Geometry check sheet. Reference: the model listing, model coordinates, mm. A direction names the side the tool comes from. Round coordinates to 2 decimals unless told otherwise and drop trailing zeros. Order: outer loops, then holes, each group sorted by start corner. A loop starts at its lowest first (then second) coordinate and runs counter-clockwise, first axis right, second up.
```python
from build123d import *

# Parameters (mm, degrees)
SKETCH2_R           = 145
SKETCH2_R_2         = 105
BOSS_EXTRUDE2_START = -50
SKETCH3_W           = 360
SKETCH3_H           = 360
SKETCH3_R           = 145
BOSS_EXTRUDE2_DEPTH = 50
FILLET4_R           = 20
SKETCH4_R           = 145
BOSS_EXTRUDE3_DEPTH = 50
SKETCH6_R           = 30
CUT_EXTRUDE1_DEPTH  = 10
CUT_EXTRUDE2_REACH  = 746.668
SKETCH7_R           = 15
CIRPATTERN1_COUNT   = 4
SKETCH9_R           = 30
CUT_EXTRUDE4_DEPTH  = 10
CUT_EXTRUDE5_REACH  = 866.02
SKETCH11_R          = 15
CIRPATTERN3_COUNT   = 4
CHAMFER1_SIZE       = 10


with BuildPart() as part:
    # Sweep-Thin1: sweep along a path in Sketch1
    with BuildLine(Plane.XY) as sweep_thin1_path:
        Line((0, 0), (-150, 0))
        ThreePointArc((-150, 0), (-333.847763109, 76.152236891), (-410, 260))
        Line((-410, 260), (-410, 410))
    # Sketch2 → Sweep-Thin1 (sweep)
    with BuildSketch(Plane(origin=(0, 0, 0), x_dir=(0, 0, -1), z_dir=(1, 0, 0))):
        Circle(SKETCH2_R)
        Circle(SKETCH2_R_2, mode=Mode.SUBTRACT)
    sweep(path=sweep_thin1_path.line)

    # Sketch3 → Boss-Extrude2 (add)
    with BuildSketch(Plane(origin=(0, 0, 0), x_dir=(0, 0, -1), z_dir=(1, 0, 0)).offset(BOSS_EXTRUDE2_START)):
        Rectangle(SKETCH3_W, SKETCH3_H)
        with Locations(Location((0, 0, 0), (0, 0, 270))):
            Circle(SKETCH3_R, mode=Mode.SUBTRACT)
    extrude(amount=BOSS_EXTRUDE2_DEPTH)

    # Fillet4
    fillet4_edges = [part.edges().sort_by_distance(p)[0] for p in [
        (-25, 180, -180),
        (-25, -180, -180),
        (-25, -180, 180),
        (-25, 180, 180),
    ]]
    fillet(fillet4_edges, radius=FILLET4_R)

    # Sketch4 → Boss-Extrude3 (add)
    with BuildSketch(Plane(origin=(0, 410, 0), x_dir=(1, 0, 0), z_dir=(0, 1, 0))):
        with BuildLine():
            Line((-255.005170931, 180), (-595.005170931, 180))
            ThreePointArc((-595.005170931, 180), (-602.076238742, 177.071067812), (-605.005170931, 170))
            Line((-605.005170931, 170), (-605.005170931, -170))
            ThreePointArc((-605.005170931, -170), (-602.076238742, -177.071067812), (-595.005170931, -180))
            Line((-595.005170931, -180), (-255.005170931, -180))
            ThreePointArc((-255.005170931, -180), (-247.934103119, -177.071067812), (-245.005170931, -170))
            Line((-245.005170931, -170), (-245.005170931, 170))
            ThreePointArc((-245.005170931, 170), (-247.934103119, 177.071067812), (-255.005170931, 180))
        make_face()
        with Locations(Location((-410, 0, 0), (0, 0, 180))):
            Circle(SKETCH4_R, mode=Mode.SUBTRACT)
    extrude(amount=-BOSS_EXTRUDE3_DEPTH)

    # Sketch6 → Cut-Extrude1 (cut)
    with BuildSketch(Plane(origin=(0, 0, 0), x_dir=(0, 0, -1), z_dir=(1, 0, 0))):
        with Locations((-130, 130)):
            Circle(SKETCH6_R)
    cut_extrude1 = extrude(amount=-CUT_EXTRUDE1_DEPTH, mode=Mode.SUBTRACT)

    # Sketch7 → Cut-Extrude2 (cut, up to next)
    with BuildSketch(Plane(origin=(-10, 0, 0), x_dir=(0, 0, -1), z_dir=(1, 0, 0)), mode=Mode.PRIVATE) as cut_extrude2_sk1:
        with Locations((-130, 130)):
            Circle(SKETCH7_R)
    cut_extrude2_tool1 = extrude(cut_extrude2_sk1.sketch, amount=-CUT_EXTRUDE2_REACH, mode=Mode.PRIVATE) & part.part
    cut_extrude2 = cut_extrude2_tool1.solids().sort_by_distance((-10, 130, 130))[0]
    add(cut_extrude2, mode=Mode.SUBTRACT)

    # CirPattern1: Cut-Extrude1, Cut-Extrude2 ×4 about axis
    cirpattern1_axis = Axis((0, 0, 0), (1, 0, 0))
    add([cut_extrude1.rotate(cirpattern1_axis, i * 360 / CIRPATTERN1_COUNT) for i in range(1, CIRPATTERN1_COUNT)], mode=Mode.SUBTRACT)
    add([cut_extrude2.rotate(cirpattern1_axis, i * 360 / CIRPATTERN1_COUNT) for i in range(1, CIRPATTERN1_COUNT)], mode=Mode.SUBTRACT)

    # Sketch9 → Cut-Extrude4 (cut)
    with BuildSketch(Plane(origin=(0, 410, 0), x_dir=(1, 0, 0), z_dir=(0, 1, 0))):
        with Locations(Location((-540, 130, 0), (0, 0, 180))):
            Circle(SKETCH9_R)
    cut_extrude4 = extrude(amount=-CUT_EXTRUDE4_DEPTH, mode=Mode.SUBTRACT)

    # Sketch11 → Cut-Extrude5 (cut, up to next)
    with BuildSketch(Plane(origin=(0, 410, 0), x_dir=(1, 0, 0), z_dir=(0, 1, 0)), mode=Mode.PRIVATE) as cut_extrude5_sk1:
        with Locations(Location((-540, 130, 0), (0, 0, 180))):
            Circle(SKETCH11_R)
    cut_extrude5_tool1 = extrude(cut_extrude5_sk1.sketch, amount=-CUT_EXTRUDE5_REACH, mode=Mode.PRIVATE) & part.part
    cut_extrude5 = cut_extrude5_tool1.solids().sort_by_distance((-540, 410, -130))[0]
    add(cut_extrude5, mode=Mode.SUBTRACT)

    # CirPattern3: Cut-Extrude4, Cut-Extrude5 ×4 about axis
    cirpattern3_axis = Axis((-410, 0, 0), (0, 1, 0))
    add([cut_extrude4.rotate(cirpattern3_axis, i * 360 / CIRPATTERN3_COUNT) for i in range(1, CIRPATTERN3_COUNT)], mode=Mode.SUBTRACT)
    add([cut_extrude5.rotate(cirpattern3_axis, i * 360 / CIRPATTERN3_COUNT) for i in range(1, CIRPATTERN3_COUNT)], mode=Mode.SUBTRACT)

    # Chamfer1
    chamfer1_edges = [part.edges().sort_by_distance(p)[0] for p in [
        (0, 0, 105),
        (-410, 410, 105),
    ]]
    chamfer(chamfer1_edges, length=CHAMFER1_SIZE)


solid = part.part
```
(1) Material ranges on line 1 (Z direction, x = -540, y = 381); line 2 (X direction, y = 374.5, z = -130); line 3 (X direction, y = 356, z = 0), recorded low to high.
Returned:
line 1: z = -180 to -145, -115 to 115, 145 to 180
line 2: x = -605.01 to -555, -525 to -295, -265 to -245.01
line 3: x = -555 to -515, -305 to -265
(2) Set-up check for faces 4 (the flat face through (-245.005, 385, 2)), 5 (the flat face through (-10, -124, -144)), 6 (the cylindrical face through (-567.712, 405.07, -141.49)): record each of +Z, -Z, +X, -X, +Y, -Y from which the full face is reachable in a straight line by a thin tool's end or side.
Returned:
face 4: +Z, -Z, +X, +Y
face 5: +X
face 6: +Y
(3) Sectioned sample at A-A, the plane z = 0. Record the cut outline in (x, y), and give its area (3 significant figures).
Returned:
outline: (-605.01, 360) - (-555, 360) - (-555, 260) arc R405 ccw to (-150, -145) - (-50, -145) - (-50, -180) - (0, -180) - (0, -115) - (-10, -105) - (-150, -105) arc R365 cw to (-515, 260) - (-515, 400) - (-525, 410) - (-605.01, 410) - close; (-305, 260) arc R155 ccw to (-150, 105) - (-10, 105) - (0, 115) - (0, 180) - (-50, 180) - (-50, 145) - (-150, 145) arc R115 cw to (-265, 260) - (-265, 360) - (-245.01, 360) - (-245.01, 410) - (-295, 410) - (-305, 400) - close
area: 63,500 mm2
(4) Depth check by flat-ended pin: P1, Ø24, axis at y = -130, z = -130, coming from the +X side; P2, Ø12, axis at x = -228, y = 9.5, coming from the +Z side; P3, Ø1, axis at y = 199.5, z = -108, coming from the +X side; P4, Ø3, axis at y = 165, z = 126.5, coming from the +X side. Enter the tip coordinate at first touch or a pass-through.
Returned:
P1: passes through
P2: stops at z = 145
P3: stops at x = -300.99
P4: stops at x = 0
(5) Sectioned sample at B-B, the plane x = -280. Give the number of separate pieces and of enclosed holes in the cut face, and give its area (3 significant figures).
Returned:
separate pieces: 3
enclosed holes: 1
area: 71,600 mm2
(6) Draft check along X on faces 1 (the flat face through (-546, 400, -116)), 2 (the conical face through (-9.4, 93.7, -48.7)), 3 (the cylindrical face through (-80.98, -31.54, -100.15)). Enter one of: released by +X, released by -X, zero draft, split by the parting line, or undercut.
Returned:
face 1: undercut
face 2: released by +X
face 3: zero draft
